For this review, take the finished solid that the model builds, in its own axes (mm). A direction names the side the tool comes from. Round coordinates to 2 decimals unless told otherwise and drop trailing zeros. Write each loop counter-clockwise with the first axis right and the second up, starting at its lowest first coordinate (ties: lowest second). Pieces come first, ordered by that corner, then holes. Notation, with made-up numbers: (87, 55.25) -> (115, 55.25) arc R23 cw to (115, 84.25) -> close; hole circle Ø1 at (73.25, 46.5). An arc over 180 degrees is marked (long way). Answer as CSV lines item,"result". Start each with the question number.
Item 1: For pin 1 Ø3 at (x, z) = (9.5, 0) entering from -Y; pin 2 Ø0.9 at (y, z) = (1.5, 11.5) entering from +X; pin 3 Ø0.9 at (y, z) = (1.5, 13) entering from +X; pin 4 Ø0.9 at (y, z) = (2, 4.5) entering from +X, all flat-tipped, find the tip position at first contact; note any pin that passes through.
Item 2: Take a section at A-A on x = 0. Give the boundary of the cut face in (y, z).
Item 3: Wall thickness on probe 1 along X at (y, z) = (2.85, -6.5); probe 2 along X at (y, z) = (1.6, 9.5); probe 3 along X at (y, z) = (1.25, 0): over which ranges is each line inside the solid? List them lowest first. Write a range as from..to.
Item 4: Machinability: for faces 1 (the cylindrical face through (-16.872, 1.479, 3.164)), 2 (the flat face through (-14.57, 1.48, -1.87)), 3 (the flat face through (-12.85, 1, 13)), which of the approach directions +Z, -Z, +X, -X, +Y, -Y give a long, thin tool a straight path to every point of the face, cutting with its end or side? Answer none if there is none.
Item 5: Take a section at B-B on z = -55. Give the boundary of the cut face in (x, y), then the cut area to 3 significant figures.
Item 6: Mouldability with a two-part tool opening along Z and no side actions: class faces 4 (the flat face through (-17.662, 1.479, -4.573)), 5 (the cylindrical face through (22.904, 1.479, -9.892)), 6 (the cylindrical face through (16.947, 1.479, 3.155)), 7 (the flat face through (5.71, 1, 13)) as +Z half, -Z half, draft (parallel to the pull), parting line (faces both ways), or undercut.
```python
from build123d import *

# Parameters (mm, degrees)
BOSS_EXTRUDE1_DEPTH = 3


with BuildPart() as part:
    # Sketch1 → Boss-Extrude1 (new body)
    with BuildSketch(Plane(origin=(0, 0, 0), x_dir=(1, 0, 0), z_dir=(0, 1, 0))):
        with BuildLine():
            Line((10.463176551, 6.170000059), (4.475348529, 63.140378143))
            ThreePointArc((4.475348529, 63.140378143), (0, 67.170000059), (-4.475348529, 63.140378143))
            Line((-4.475348529, 63.140378143), (-10.463176551, 6.170000059))
            Line((-10.463176551, 6.170000059), (-10.594086082, 6.333950269))
            ThreePointArc((-10.594086082, 6.333950269), (-12.700318865, 7.010801248), (-14.141740272, 5.332513992))
            Line((-14.141740272, 5.332513992), (-15.012961009, -1.682423602))
            ThreePointArc((-15.012961009, -1.682423602), (-16.909521943, -3.15994065), (-18.387038991, -1.263379717))
            Line((-18.387038991, -1.263379717), (-16.916878018, 10.574134051))
            Line((-16.916878018, 10.574134051), (-18.076495252, 10.884852553))
            ThreePointArc((-18.076495252, 10.884852553), (-22.84818786, 9.93570388), (-25, 5.572260508))
            Line((-25, 5.572260508), (-25, 0.469626677))
            ThreePointArc((-25, 0.469626677), (-24.758369054, -4.440028009), (-24.035811635, -9.302229714))
            Line((-24.035811635, -9.302229714), (-23.801666433, -10.47718558))
            ThreePointArc((-23.801666433, -10.47718558), (-22.069368276, -13.365612971), (-18.89808527, -14.499999941))
            Line((-18.89808527, -14.499999941), (-12.85, -14.499999941))
            Line((-12.85, -14.499999941), (-12.85, -10.549999941))
            ThreePointArc((-12.85, -10.549999941), (-9.28, -6.979999941), (-5.71, -10.549999941))
            Line((-5.71, -10.549999941), (-5.71, -14.499999941))
            Line((-5.71, -14.499999941), (-1.500000059, -14.499999941))
            Line((-1.500000059, -14.499999941), (-1.500000059, 0))
            ThreePointArc((-1.500000059, 0), (0, 1.500000059), (1.500000059, 0))
            Line((1.500000059, 0), (1.500000059, -14.499999941))
            Line((1.500000059, -14.499999941), (5.71, -14.499999941))
            Line((5.71, -14.499999941), (5.71, -10.549999941))
            ThreePointArc((5.71, -10.549999941), (9.28, -6.979999941), (12.85, -10.549999941))
            Line((12.85, -10.549999941), (12.85, -14.499999941))
            Line((12.85, -14.499999941), (18.89808527, -14.499999941))
            ThreePointArc((18.89808527, -14.499999941), (22.069368276, -13.365612971), (23.801666433, -10.47718558))
            Line((23.801666433, -10.47718558), (24.035811635, -9.302229714))
            ThreePointArc((24.035811635, -9.302229714), (24.758369054, -4.440028009), (25, 0.469626677))
            Line((25, 0.469626677), (25, 5.572260508))
            ThreePointArc((25, 5.572260508), (22.84818786, 9.93570388), (18.076495252, 10.884852553))
            Line((18.076495252, 10.884852553), (16.916878018, 10.574134051))
            Line((16.916878018, 10.574134051), (18.387038991, -1.263379717))
            ThreePointArc((18.387038991, -1.263379717), (16.909521943, -3.15994065), (15.012961009, -1.682423602))
            Line((15.012961009, -1.682423602), (14.141740272, 5.332513992))
            ThreePointArc((14.141740272, 5.332513992), (12.700318865, 7.010801248), (10.594086082, 6.333950269))
            Line((10.594086082, 6.333950269), (10.463176551, 6.170000059))
        make_face()
    extrude(amount=BOSS_EXTRUDE1_DEPTH)


solid = part.part
```
Output values:
1,pin 1,"stops at y = 0"
1,pin 2,"stops at x = 23.65"
1,pin 3,"stops at x = 22.86"
1,pin 4,"stops at x = 24.8"
2,outline,"(0, -67.17) -> (3, -67.17) -> (3, -1.5) -> (0, -1.5) -> close"
3,probe 1,"x = -24.92..-17.42, -13.57..-10.74, -10.43..10.43, 10.74..13.57, 17.42..24.92"
3,probe 2,"x = -24..-12.69, -5.87..-1.5, 1.5..5.87, 12.69..24"
3,probe 3,"x = -25..-18.23, -14.8..-1.5, 1.5..14.8, 18.23..25"
4,face 1,"+Y, -Y"
4,face 2,"-Z, +Y, -Y"
4,face 3,"+Z, +Y, -Y"
5,outline,"(-5.33, 0) -> (5.33, 0) -> (5.33, 3) -> (-5.33, 3) -> close"
5,area,"32.0 mm^2"
6,face 4,"undercut"
6,face 5,"-Z half"
6,face 6,"undercut"
6,face 7,"draft"
